CAD build for the part. Positions are in the model's coordinates, mm. Face numbers are marked on the shaded views. A direction names the side the tool comes from. Give positions to 0.01 mm unless a question says otherwise; leave off trailing zeros. Order: outer loops, then holes, each group sorted by start corner. A loop starts at its lowest first (then second) coordinate and runs counter-clockwise, first axis right, second up.
Item 1: Band-saw the part on A-A on z = 16.5. Give the cut face in (x, y), plus the area to 3 significant figures.
Item 2: Flat gauge pins, fed straight in: P1, Ø9.5, axis at x = -9, z = 6.5, coming from the +Y side; P2, Ø2, axis at x = 7, y = 8, coming from the +Z side; P3, Ø6, axis at y = 9.5, z = 9.5, coming from the +X side; P4, Ø3, axis at x = 4.86, z = 16.5, coming from the +Y side. Where does each tip first touch, or does it go through?
Item 3: Band-saw the part on D-D on z = 11.5. Give the cut face in (x, y).
Item 4: Which spindle directions (+Z, -Z, +X, -X, +Y, -Y) get a long thin tool onto all of the face, cutting with end or side? Do the marked faces 1, 2 and 3. Say none if no direction does.
Item 5: Band-saw the part on C-C on z = 0. Give the cut face in (x, y), plus the area to 3 significant figures.
Item 6: Band-saw the part on B-B on x = 1. Give the cut face in (y, z).
Item 7: Wall check: L1, parallel to Y at x = 1.4, z = 0; L2, parallel to X at y = 2.15, z = 16.5; L3, parallel to X at y = 1, z = 16.5. Give the ranges that are in metal, low to high.
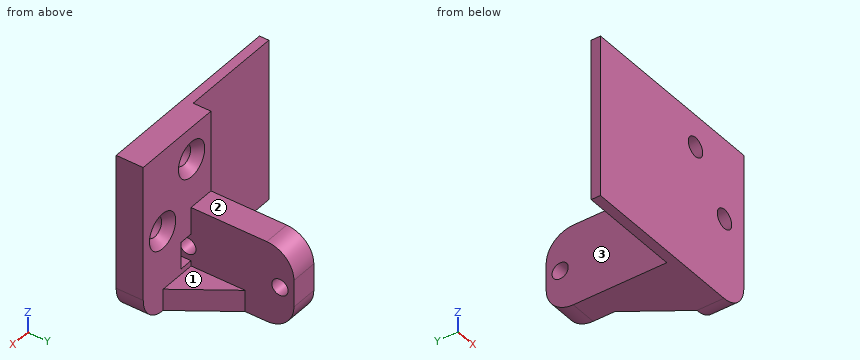
```python
from build123d import *

# Parameters (mm, degrees)
SKETCH_1_W                = 15
SKETCH_1_H                = 24
SKETCH_1_R                = 1.5
EXTRUDE_1_DEPTH           = 5
SKETCH_2_W                = 30
SKETCH_2_H                = 1.720004632
EXTRUDE_2_DEPTH           = 19
EXTRUDE_5_DEPTH           = 5
SKETCH_7_W                = 2.5
SKETCH_7_H                = 5
CUT_EXTRUDE_1_DEPTH       = 3
FILLET_1_R                = 5
HOLE_WIZARD_1_D           = 3.6
HOLE_WIZARD_1_CSINK_D     = 6.6
HOLE_WIZARD_1_CSINK_ANGLE = 90
RIB_1_REACH               = 44.86
SKETCH_10_WALL_W          = 99.927031582
SKETCH_10_WALL_H          = 4


with BuildPart() as part:
    # 草图1 → 凸台-拉伸1 (new body)
    with BuildSketch(Plane(origin=(0, 0, 0), x_dir=(0, 0, -1), z_dir=(1, 0, 0))):
        with Locations((0, 12)):
            Rectangle(SKETCH_1_W, SKETCH_1_H)
        with Locations((0, 4.420004632)):
            Circle(SKETCH_1_R, mode=Mode.SUBTRACT)
        with Locations((0, 21.420004632)):
            Circle(SKETCH_1_R, mode=Mode.SUBTRACT)
    extrude(amount=EXTRUDE_1_DEPTH)

    # 草图2 → 凸台-拉伸2 (add)
    with BuildSketch(Plane.ZY):
        with Locations((7.5, 0.860002316)):
            Rectangle(SKETCH_2_W, SKETCH_2_H)
    extrude(amount=EXTRUDE_2_DEPTH)

    # 草图4 → 凸台-拉伸5 (add)
    with BuildSketch(Plane(origin=(0, 0, 0), x_dir=(1, 0, 0), z_dir=(0, 1, 0))):
        Polygon((5, 7.5), (17, 7.5), (17, -22.5), (0, -22.5), (0, -7.5), (5, -7.5), align=None)
    extrude(amount=EXTRUDE_5_DEPTH)

    # 草图7 → 切除-拉伸1 (cut)
    with BuildSketch(Plane(origin=(0, 5, 0), x_dir=(1, 0, 0), z_dir=(0, 1, 0))):
        with Locations((6.25, 0)):
            Rectangle(SKETCH_7_W, SKETCH_7_H)
    extrude(amount=-CUT_EXTRUDE_1_DEPTH, mode=Mode.SUBTRACT)

    # 圆角1
    fillet_1_edges = [part.edges().sort_by_distance(p)[0] for p in [
        (17, 2.5, -7.5),
        (2.5, 24, 7.5),
        (2.5, 24, -7.5),
    ]]
    fillet(fillet_1_edges, radius=FILLET_1_R)

    # 打孔尺寸(%根据十字)槽半沉头木螺钉的类型1 (through all)
    with Locations(Plane(origin=(0, 5, 0), x_dir=(1, 0, 0), z_dir=(0, 1, 0))):
        with Locations((4.857142857, -16.5), (12.142857143, -7.5)):
            CounterSinkHole(HOLE_WIZARD_1_D / 2, HOLE_WIZARD_1_CSINK_D / 2, counter_sink_angle=HOLE_WIZARD_1_CSINK_ANGLE)

    # 草图10 wall → 筋1 (add, up to next)
    with BuildSketch(Plane(origin=(8.5, 10, -7.5), x_dir=(-0.573462344363, 0.819231920519, 0), z_dir=(0.819231920519, 0.573462344363, 0)), mode=Mode.PRIVATE) as rib_1_sk1:
        with Locations((0, 2)):
            Rectangle(SKETCH_10_WALL_W, SKETCH_10_WALL_H)
    rib_1_tool1 = extrude(rib_1_sk1.sketch, amount=-RIB_1_REACH, mode=Mode.PRIVATE) - part.part
    add(rib_1_tool1.solids().sort_by_distance((8.5, 10, -7.5))[0])


solid = part.part
```
The answers:
1. outline: (-19, 0) - (3.06, 0) - (3.06, 3.5) - (1.56, 5) - (0, 5) - (0, 1.72) - (-19, 1.72) - close; (6.66, 0) - (17, 0) - (17, 5) - (8.16, 5) - (6.66, 3.5) - close
1. area: 97.4 mm2
2. P1: stops at y = 1.72
2. P2: stops at z = -3.5
2. P3: stops at x = 5
2. P4: passes through
3. outline: (-19, 0) - (17, 0) - (17, 5) - (0, 5) - (0, 1.72) - (-19, 1.72) - close
4. face 1: +Z, +X, +Y
4. face 2: +Z, +X, -X, +Y
4. face 3: +Z, -Z, -X, +Y
5. outline: (-19, 0) - (17, 0) - (17, 5) - (7.5, 5) - (7.5, 2) - (5, 2) - (5, 2.92) - (0, 2.92) - (0, 1.72) - (-19, 1.72) - close; (0, 5.92) - (5, 5.92) - (5, 19.92) - (0, 19.92) - close; (0, 22.92) - (5, 22.92) - (5, 24) - (0, 24) - close
5. area: 175 mm2
6. outline: (0, -7.5) - (19, -7.5) arc R5 ccw to (24, -2.5) - (24, 2.5) arc R5 ccw to (19, 7.5) - (5, 7.5) - (5, 22.5) - (0, 22.5) - close; hole circle Ø3 at (4.42, 0); hole circle Ø3 at (21.42, 0)
7. L1: y = 0 to 2.92, 5.92 to 19.92, 22.92 to 24
7. L2: x = 0 to 3.06, 6.66 to 17
7. L3: x = -19 to 3.06, 6.66 to 17
